Verification items for the finished model (mm, model axes). A direction names the side the tool comes from. Give positions to 0.01 mm unless a question says otherwise; leave off trailing zeros. Order: outer loops, then holes, each group sorted by start corner. A loop starts at its lowest first (then second) coordinate and runs counter-clockwise, first axis right, second up. Notation, with made-up numbers: M 40,-18.5 L 79,-18.5 A9 cw 79,-14.5 Z; hole C -13,47.5 d11. An arc over 180 degrees is marked long. Answer as a JSON object with one key per item and string values.
```python
from build123d import *

# Parameters (mm, degrees)
SZKIC1_R                              = 10
DODANIE_WYCI_GNI_CIE1_DEPTH           = 10
DODANIE_WYCI_GNI_CIE2_DEPTH           = 7
SZKIC3_W                              = 26
SZKIC3_H                              = 7
DODANIE_WYCI_GNI_CIE3_DEPTH           = 5
DODANIE_WYCI_GNI_CIE4_DEPTH           = 7
DODANIE_WYCI_GNI_CIE5_DEPTH           = 21
ZAOKR_GLENIE2_R                       = 0.5
SZKIC8_W                              = 0.687995553
SZKIC8_H                              = 26
DODANIE_WYCI_GNI_CIE6_DEPTH           = 20
DODANIE_WYCI_GNI_CIE6_TAPER           = -1
DODANIE_WYCI_GNI_CIE6_OTHER_WAY_DEPTH = 10


with BuildPart() as part:
    # Szkic1 → Dodanie-wyciągnięcie1 (new body)
    with BuildSketch(Plane.XY):
        with BuildLine():
            Line((-10.593939394, 20.448484848), (-10.593939394, -7.551515152))
            Line((-10.593939394, -7.551515152), (-28.593939394, -7.551515152))
            ThreePointArc((-28.593939394, -7.551515152), (-42.593939394, 6.448484848), (-28.593939394, 20.448484848))
            Line((-28.593939394, 20.448484848), (-10.593939394, 20.448484848))
        make_face()
        with Locations((-28.593939394, 6.448484848)):
            Circle(SZKIC1_R, mode=Mode.SUBTRACT)
    extrude(amount=DODANIE_WYCI_GNI_CIE1_DEPTH)

    # Szkic2 → Dodanie-wyciągnięcie2 (add)
    with BuildSketch(Plane(origin=(-10.593939394, 0, 0), x_dir=(0, 0, -1), z_dir=(1, 0, 0))):
        Polygon((-10, 20.448484848), (-18, 20.448484848), (-18, -7.551515152), (-10, -7.551515152), (0, -7.551515152), (8, -7.551515152), (8, 20.448484848), (0, 20.448484848), align=None)
    extrude(amount=DODANIE_WYCI_GNI_CIE2_DEPTH)

    # Szkic3 → Dodanie-wyciągnięcie3 (add)
    with BuildSketch(Plane(origin=(-3.593939394, 0, 0), x_dir=(0, 0, -1), z_dir=(1, 0, 0))):
        with Locations((-5, -4.051515152)):
            Rectangle(SZKIC3_W, SZKIC3_H)
    extrude(amount=DODANIE_WYCI_GNI_CIE3_DEPTH)

    # Szkic4 → Dodanie-wyciągnięcie4 (add)
    with BuildSketch(Plane(origin=(0, -0.551515152, 0), x_dir=(1, 0, 0), z_dir=(0, 1, 0))):
        with BuildLine():
            Line((1.406060606, -18), (1.406060606, 8))
            Line((1.406060606, 8), (31.406060606, 4))
            Line((31.406060606, 4), (31.406060606, 0))
            Line((31.406060606, 0), (23.406060606, 0))
            ThreePointArc((23.406060606, 0), (18.406060606, -5), (23.406060606, -10))
            Line((23.406060606, -10), (31.406060606, -10))
            Line((31.406060606, -10), (31.406060606, -14))
            Line((31.406060606, -14), (1.406060606, -18))
        make_face()
    extrude(amount=-DODANIE_WYCI_GNI_CIE4_DEPTH)

    # Szkic5 → Dodanie-wyciągnięcie5 (add)
    with BuildSketch(Plane(origin=(0, -0.551515152, 0), x_dir=(1, 0, 0), z_dir=(0, 1, 0))):
        with BuildLine():
            Line((-3.593939394, 8.043944751), (-3.593939394, 5.043944751))
            ThreePointArc((-3.593939394, 5.043944751), (6.450005357, -5), (-3.593939394, -15.043944751))
            Line((-3.593939394, -15.043944751), (-3.593939394, -18.043944751))
            ThreePointArc((-3.593939394, -18.043944751), (9.450005357, -5), (-3.593939394, 8.043944751))
        make_face()
    extrude(amount=DODANIE_WYCI_GNI_CIE5_DEPTH)

    # Zaokrąglenie2
    zaokr_glenie2_edges = [part.edges().sort_by_distance(p)[0] for p in [
        (-3.593939394, 9.948484848, 15.043944751),
    ]]
    fillet(zaokr_glenie2_edges, radius=ZAOKR_GLENIE2_R)

    # Szkic8 → Dodanie-wyciągnięcie6 (add)
    with BuildSketch(Plane.XZ.offset(7.551515152)):
        with Locations((-4.937937171, 5)):
            Rectangle(SZKIC8_W, SZKIC8_H)
    extrude(amount=DODANIE_WYCI_GNI_CIE6_DEPTH, taper=DODANIE_WYCI_GNI_CIE6_TAPER)

    # Szkic8 → Dodanie-wyciągnięcie6 other way (add)
    with BuildSketch(Plane.XZ.offset(7.551515152)):
        with Locations((-4.937937171, 5)):
            Rectangle(SZKIC8_W, SZKIC8_H)
    extrude(amount=-DODANIE_WYCI_GNI_CIE6_OTHER_WAY_DEPTH)


solid = part.part
```
Q1. Section check D-D on x = -21.5. Record the cut outline in (y, z), then the cut area to 3 significant figures.
Resolved:
{"outline": "M -7.55,0 L -0.6,0 L -0.6,10 L -7.55,10 Z; M 13.5,0 L 20.45,0 L 20.45,10 L 13.5,10 Z", "area": "139 mm²"}
Q2. Tool access check on faces 1 (the face through (9.447, 9.801, 5.287)), 2 (the face through (27, -4, 10)), 3 (the face through (-19, 13, 0)), 4 (the face through (6.44, 9.8, 4.52)), 5 (the face through (-10.594, 7, 14)). Record the directions out of +Z, -Z, +X, -X, +Y, -Y that give a thin tool (end or side, any length) a straight path to the whole face; none if there is none.
Resolved:
{"face 1": "+X, +Y", "face 2": "+X, +Y, -Y", "face 3": "-Z, -X, +Y, -Y", "face 4": "+Y", "face 5": "+Z, -X, +Y, -Y"}
Q3. Section check C-C on y = -5. Record the cut outline in (x, z), then the cut area to 3 significant figures.
Resolved:
{"outline": "M -36.65,0 L -10.59,0 L -10.59,-8 L 1.41,-8 L 31.41,-4 L 31.41,0 L 23.41,0 A5 cw 23.41,10 L 31.41,10 L 31.41,14 L 1.41,18 L -10.59,18 L -10.59,10 L -36.65,10 Z", "area": "1,110 mm²"}
Q4. Release check for a two-part mould opening along X. For faces 6 (the face through (-42.59, 6.14, 4.93)), 7 (the face through (0, -0.552, 5)), 8 (the face through (15, -0.552, 5)) record: +X half, -X half, draft (parallel to the pull), parting line (faces both ways), or undercut.
Resolved:
{"face 6": "-X half", "face 7": "undercut", "face 8": "draft"}
Q5. Gauge pin test, flat ends, axial feed: pin 1 Ø8 at (x, y) = (20, -9.5) entering from -Z; pin 2 Ø2 at (x, y) = (28.5, -5.5) entering from -Z; pin 3 Ø6 at (y, z) = (9.5, 7) entering from +X. Record the tip position at first contact, or that the pin passes through.
Resolved:
{"pin 1": "stops at z = -5.99", "pin 2": "stops at z = -4.52", "pin 3": "stops at x = 9.45"}
Q6. Section check A-A on y = 5.5. Record the cut outline in (x, z).
Resolved:
{"outline": "M -42.56,0 L -38.55,0 L -38.55,10 L -42.56,10 Z; M -18.64,0 L -10.59,0 L -10.59,-8 L -3.59,-8 L -3.59,-8.04 A13.04 ccw -3.59,18.04 L -3.59,18 L -10.59,18 L -10.59,10 L -18.64,10 Z; hole M -3.59,-5.04 A10.04 ccw -3.07,15.03 A0.5 ccw -3.59,14.53 Z"}
Q7. Section check B-B on x = -35.5. Record the cut outline in (y, z).
Resolved:
{"outline": "M -5.73,0 L -0.78,0 L -0.78,10 L -5.73,10 Z; M 13.68,0 L 18.63,0 L 18.63,10 L 13.68,10 Z"}
Q8. Material ranges on L1, parallel to X at y = 7.5, z = 9.5; L2, parallel to X at y = 10, z = 7; L3, parallel to Y at x = -12, z = 3.25, recorded low to high.
Resolved:
{"L1": "x = -42.55 to -38.54, -18.65 to -3.59, 5.39 to 8.65", "L2": "x = -42.14 to -37.94, -19.25 to -3.59, 6.25 to 9.3", "L3": "y = -7.55 to 20.45"}
